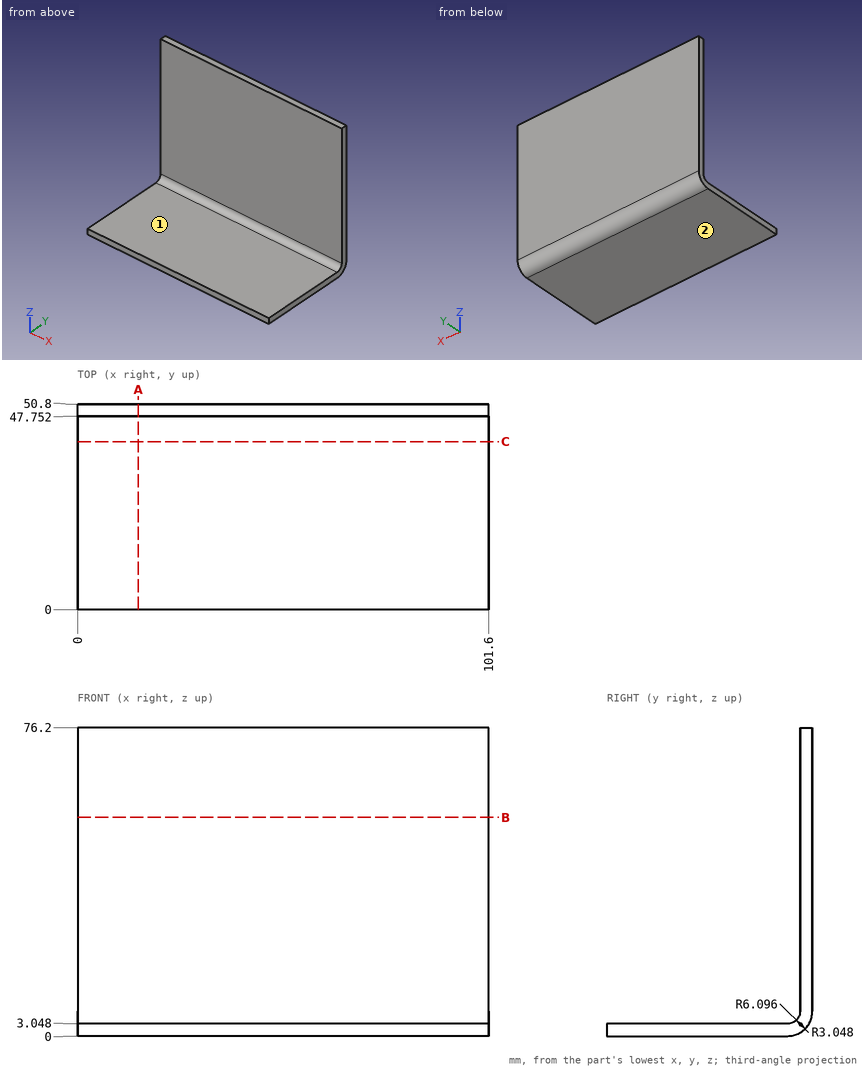
Job drawing, mm, ordinate dimensions from the low corner. One solid piece. A direction names the side the tool comes from. Give positions to 0.01 mm unless a question says otherwise; leave off trailing zeros. Order: outer loops, then holes, each group sorted by start corner. A loop starts at its lowest first (then second) coordinate and runs counter-clockwise, first axis right, second up. Notation, with made-up numbers: M 12,-14 L 55,-14 A31 cw 55,15 Z; hole C 4,17.5 d11. An arc over 180 degrees is marked long. Return JSON: item names as keys, results as strings.
Q1. 3-axis set-ups, long thin cutter, end or side, ignore diameter. For the marked faces 1 and 2: which of +Z, -Z, +X, -X, +Y, -Y reach the whole face in a straight line?
Answer list:
{"face 1": "+Z, +X, -X, -Y", "face 2": "-Z, +X, -X, +Y, -Y"}
Q2. Band-saw the part on B-B (z = 54). Give the cut face in (x, y).
Answer list:
{"outline": "M 0,47.75 L 101.6,47.75 L 101.6,50.8 L 0,50.8 Z"}
Q3. Band-saw the part on A-A (x = 15). Give the cut face in (y, z), then the cut area to 3 significant figures.
Answer list:
{"outline": "M 0,0 L 44.7,0 A6.1 ccw 50.8,6.1 L 50.8,76.2 L 47.75,76.2 L 47.75,6.1 A3.05 cw 44.7,3.05 L 0,3.05 Z", "area": "372 mm^2"}
Q4. Wall check: probe 1 along Y at (x, z) = (18.5, 67); probe 2 along Z at (x, y) = (58, 24.5); probe 3 along Y at (x, z) = (63, 4.5). Give the ranges that are in metal, low to high. Write a range as from..to.
Answer list:
{"probe 1": "y = 47.75..50.8", "probe 2": "z = 0..3.05", "probe 3": "y = 47.3..50.59"}
Q5. Band-saw the part on C-C (y = 41.5). Give the cut face in (x, z).
Answer list:
{"outline": "M 0,0 L 101.6,0 L 101.6,3.05 L 0,3.05 Z"}
Q6. Flat gauge pins, fed straight in: pin 1 (1.5 mm diameter, centred on x = 26, y = 25.5, fed in from -Z); pin 2 (1.5 mm diameter, centred on x = 15.5, y = 36.5, fed in from +Z); pin 3 (21 mm diameter, centred on x = 46, z = 38, fed in from -Y). Where does each tip first touch, or does it go through?
Answer list:
{"pin 1": "stops at z = 0", "pin 2": "stops at z = 3.05", "pin 3": "stops at y = 47.75"}
